Check sheet for the modelled part. Datum: model origin and axes. Units: mm. A direction names the side the tool comes from. Give positions to 0.01 mm unless a question says otherwise; leave off trailing zeros. Write each loop counter-clockwise with the first axis right and the second up, starting at its lowest first coordinate (ties: lowest second). Pieces come first, ordered by that corner, then holes. Notation, with made-up numbers: (58, 40) - (110, 40) arc R10 ccw to (110, 59) - close; hole circle Ø2 at (56, 41.5). An arc over 180 degrees is marked (long way). Return JSON: item names as keys, results as strings. Group by question number.
```python
from build123d import *

# Parameters (mm, degrees)
F0_R     = 5
F0_R_2   = 10
F1_DEPTH = 25


with BuildPart() as f1:
    # F0 (on Top) → F1 (new body)
    with BuildSketch(Plane.XY):
        with BuildLine():
            ThreePointArc((-33.198925, -40.524198), (-30.269993, -47.595265), (-23.198925, -50.524198))
            Line((-23.198925, -50.524198), (26.801075, -50.524198))
            ThreePointArc((26.801075, -50.524198), (33.872142, -47.595265), (36.801075, -40.524198))
            ThreePointArc((36.801075, -40.524198), (33.872142, -33.45313), (26.801075, -30.524198))
            Line((26.801075, -30.524198), (-8.198925, -30.524198))
            ThreePointArc((-8.198925, -30.524198), (-15.269993, -27.595265), (-18.198925, -20.524198))
            Line((-18.198925, -20.524198), (-18.198925, -19.158835))
            Line((-18.198925, -19.158835), (-18.198925, -15.524198))
            ThreePointArc((-18.198925, -15.524198), (-17.143197, -11.052062), (-14.198925, -7.524198))
            ThreePointArc((-14.198925, -7.524198), (-9.782518, -2.232401), (-8.198925, 4.475802))
            ThreePointArc((-8.198925, 4.475802), (-12.592324, 15.082404), (-23.198925, 19.475802))
            ThreePointArc((-23.198925, 19.475802), (-33.805527, 15.082404), (-38.198925, 4.475802))
            ThreePointArc((-38.198925, 4.475802), (-36.615333, -2.232401), (-32.198925, -7.524198))
            ThreePointArc((-32.198925, -7.524198), (-29.254653, -11.052062), (-28.198925, -15.524198))
            Line((-28.198925, -15.524198), (-28.198925, -19.158835))
            Line((-28.198925, -19.158835), (-28.198925, -27.295441))
            ThreePointArc((-28.198925, -27.295441), (-28.844782, -30.830975), (-30.698925, -33.909819))
            ThreePointArc((-30.698925, -33.909819), (-32.553069, -36.988664), (-33.198925, -40.524198))
        make_face()
        with Locations((-23.198925, -40.524198)):
            Circle(F0_R, mode=Mode.SUBTRACT)
        with Locations((26.801075, -40.524198)):
            Circle(F0_R, mode=Mode.SUBTRACT)
        with Locations((-23.198925, 4.475802)):
            Circle(F0_R_2, mode=Mode.SUBTRACT)
    extrude(amount=F1_DEPTH)


solid = f1.part
```
Item 1: Mould release check, pull along Y, two halves, no side actions. Record for faces 1 (the face through (1, -50.524, 12)), 2 (the face through (-10, -31, 25)), 3 (the face through (-18.43, -39.02, 12.32)): +Y half, -Y half, draft (parallel to the pull), parting line (faces both ways), or undercut.
Item 2: Section check B-B on z = 18. Record the cut outline in (x, y).
Item 3: Material ranges on line 1 along Y through (x, z) = (-32, 15.5); line 2 along X through (y, z) = (-41, 20.25); line 3 along X through (y, z) = (-41.5, 21.5), recorded low to high. Write a range as from..to.
Item 4: Depth check by flat-ended pin: pin 1 (5.5 mm diameter, centred on y = -19, z = 9, fed in from +X); pin 2 (7.5 mm diameter, centred on x = 1, z = 6.5, fed in from +Y); pin 3 (6 mm diameter, centred on x = -23.2, y = -40.52, fed in from +Z); pin 4 (8 mm diameter, centred on y = -14, z = 6, fed in from -X). Enter the tip coordinate at first touch or a pass-through.
Item 5: Section check A-A on x = -20.5. Record the cut outline in (y, z).
Item 6: Section check C-C on y = 12. Record the cut outline in (x, z).
Item 7: Access from +Z, -Z, +X, -X, +Y, -Y to the whole of each face (thin tool, end or side, straight path). Record for faces 4 (the face through (-29.284, -10.994, 12.325)), 5 (the face through (-17.17, -11.11, 12.32)), 6 (the face through (10, -30.524, 12)), 7 (the face through (-33.19, 4.92, 12.32)), 8 (the face through (-10, -31, 0)).
Item 8: Section check D-D on x = -10. Record the cut outline in (y, z).
Reply:
{
 "1": {"face 1": "-Y half", "face 2": "draft", "face 3": "undercut"},
 "2": {"outline": "(-38.2, 4.48) arc R15 ccw to (-32.2, -7.52) arc R10 cw to (-28.2, -15.52) - (-28.2, -27.3) arc R10 cw to (-30.7, -33.91) arc R10 ccw to (-33.2, -40.52) arc R10 ccw to (-23.2, -50.52) - (26.8, -50.52) arc R10 ccw to (36.8, -40.52) arc R10 ccw to (26.8, -30.52) - (-8.2, -30.52) arc R10 cw to (-18.2, -20.52) - (-18.2, -15.52) arc R10 cw to (-14.2, -7.52) arc R15 ccw to (-8.2, 4.48) arc R15 ccw to (-23.2, 19.48) arc R15 ccw to start; hole circle Ø20 at (-23.2, 4.48); hole circle Ø10 at (-23.2, -40.52); hole circle Ø10 at (26.8, -40.52)"},
 "3": {"line 1": "-45.27..-35.78, -7.68..-0.27, 9.22..16.62", "line 2": "-33.19..-28.18, -18.22..21.82, 31.78..36.79", "line 3": "-33.15..-28.1, -18.3..21.9, 31.7..36.75"},
 "4": {"pin 1": "x = -18.12", "pin 2": "y = -30.52", "pin 3": "through", "pin 4": "x = -29.86"},
 "5": {"outline": "(-50.52, 0) - (-44.73, 0) - (-44.73, 25) - (-50.52, 25) - close; (-36.32, 0) - (-5.15, 0) - (-5.15, 25) - (-36.32, 25) - close; (14.1, 0) - (19.23, 0) - (19.23, 25) - (14.1, 25) - close"},
 "6": {"outline": "(-36.18, 0) - (-29.79, 0) - (-29.79, 25) - (-36.18, 25) - close; (-16.61, 0) - (-10.22, 0) - (-10.22, 25) - (-16.61, 25) - close"},
 "7": {"face 4": "+Z, -Z, -X", "face 5": "+Z, -Z, +X", "face 6": "+Z, -Z, +X, +Y", "face 7": "+Z, -Z", "face 8": "-Z, +X, -X, +Y, -Y"},
 "8": {"outline": "(-50.52, 0) - (-30.36, 0) - (-30.36, 25) - (-50.52, 25) - close; (-2.65, 0) - (11.6, 0) - (11.6, 25) - (-2.65, 25) - close"}
}
